```python
from build123d import *

# Parameters (mm, degrees)
BOSS_EXTRUDE1_DEPTH      = 12.7
BOSS_EXTRUDE1_DEPTH_BACK = 19.878167
SKETCH1_W                = 76.2
SKETCH1_H                = 25.4
CUT_EXTRUDE1_DEPTH       = 50.919049703
SKETCH4_R                = 7.9375
BOSS_EXTRUDE2_DEPTH      = 76.2
BOSS_EXTRUDE3_DEPTH      = 10


with BuildPart() as part:
    # Sketch1 → Boss-Extrude1 (new, two sides: drawn at the far end of the back side and taken through both)
    with BuildSketch(Plane.XY.offset(-BOSS_EXTRUDE1_DEPTH_BACK)):
        Rectangle(SKETCH1_W, SKETCH1_H)
    extrude(amount=BOSS_EXTRUDE1_DEPTH + BOSS_EXTRUDE1_DEPTH_BACK)

    # Sketch2 → Cut-Extrude1 (cut, through all)
    with BuildSketch(Plane.XZ.offset(12.7)):
        Polygon((33.097822487, -3.5890835), (28.095644974, -19.878167), (30.299971912, -19.878167), (38.1, -19.878167), (38.1, -5.125190787), align=None)
        Polygon((38.1, 12.7), (33.097822487, -3.5890835), (38.1, -5.125190787), align=None)
        with BuildLine():
            Line((28.095644974, -19.878167), (-38.1, -19.878167))
            Line((-38.1, -19.878167), (-38.1, 2.7))
            Line((-38.1, 2.7), (-9.105646135, 2.7))
            add(Edge.make_bspline(
                [(28.095644974, -19.878167), (23.262476233, -19.878167), (13.759725723, -18.38827049), (5.19295176, 1.21010349), (-4.185142014, 2.7), (-9.105646135, 2.7)],
                knots=[0, 0, 0, 0, 0.311689084, 0.688310916, 1, 1, 1, 1], degree=3))
        make_face()
    extrude(amount=-CUT_EXTRUDE1_DEPTH, mode=Mode.SUBTRACT)

    # Sketch4 → Boss-Extrude2 (add)
    with BuildSketch(Plane(origin=(31.252760971, 0, -9.59733911), x_dir=(-0.2935578385035089, 0, -0.95594131381228), z_dir=(0.95594131381228, 0, -0.2935578385035089))):
        with Locations((-2.530674188, 0)):
            Circle(SKETCH4_R)
    extrude(amount=BOSS_EXTRUDE2_DEPTH)

    # Sketch5 → Boss-Extrude3 (add)
    with BuildSketch(Plane(origin=(0, 0, 2.7), x_dir=(-1, 0, 0), z_dir=(0, 0, -1))):
        Polygon((9.105646135, -12.7), (28.322642206, -26.407350084), (38.1, -12.7), align=None)
        Polygon((38.1, -12.7), (56.217643925, 12.7), (38.1, 12.7), align=None)
        Polygon((16.319736518, -17.845760662), (21.108551823, -21.261589422), (19.992545993, -32.851753107), (5.724357418, -22.674353105), align=None)
    extrude(amount=-BOSS_EXTRUDE3_DEPTH)


solid = part.part
```
For this review, take the finished solid that the model builds, in its own axes (mm). A direction names the side the tool comes from. Give positions to 0.01 mm unless a question says otherwise; leave off trailing zeros. Order: outer loops, then holes, each group sorted by start corner. A loop starts at its lowest first (then second) coordinate and runs counter-clockwise, first axis right, second up.
1) For faces 4 (the face through (-24.67, -23.8, 7.63)), 5 (the face through (-10.948, -20.294, 7.63)), 6 (the face through (34.28, -3, 0.26)), list the 3-axis set-ups (+Z, -Z, +X, -X, +Y, -Y) from which the entire face can be reached by the end or side of a thin tool; tool diameter is ignored.
2) Wall thickness on line 1 (Z direction, x = -29.5, y = -16); line 2 (Y direction, x = 4, z = 2); line 3 (Z direction, x = 22, y = 7.5): over which ranges is each line inside the solid? List them lowest first.
3) Take a section at B-B (y = -30). Give the boundary of the cut face in (x, z).
4) Insertion check: pin 1 (1 mm diameter, centred on y = -7.5, z = -15, fed in from -X); pin 2 (10 mm diameter, centred on x = -27.5, y = -22, fed in from -Z); pin 3 (8 mm diameter, centred on y = -16.5, z = -22, fed in from -X); pin 4 (2 mm diameter, centred on x = 28, y = 3, fed in from -Z). Each pin has a flat end and moves straight along its axis. Give the tip position at first contact, or say it passes through.
5) The part is to be moulded in two halves that separate along X. For faces 1 (the face through (-20.558, -26.976, 7.63)), 2 (the face through (1, 12.7, 3)), 3 (the face through (-12.662, -15.237, 7.63)), say which applies: released by +X, released by -X, zero draft, split by the parting line, or undercut.
6) Take a section at A-A (z = 4.5). Give the boundary of the cut face in (x, y).
7) Take a section at C-C (x = -33). Give the boundary of the cut face in (y, z), then the cut area to 4 significant figures.
Derived:
1. face 4: +Z, -Z, -Y
1. face 5: +Z, -Z, +X
1. face 6: none
2. line 1: z = 2.7 to 12.7
2. line 2: y = -12.7 to 12.7
2. line 3: z = -19.33 to 12.7
3. outline: (-20.27, 2.7) - (-15.99, 2.7) - (-15.99, 12.7) - (-20.27, 12.7) - close
4. pin 1: stops at x = 13.83
4. pin 2: stops at z = 2.7
4. pin 3: passes through
4. pin 4: stops at z = -19.88
5. face 1: undercut
5. face 2: zero draft
5. face 3: released by +X
6. outline: (-56.22, 12.7) - (-28.32, -26.41) - (-21.11, -21.26) - (-19.99, -32.85) - (-5.72, -22.67) - (-16.32, -17.85) - (-9.11, -12.7) - (35.58, -12.7) - (35.58, 12.7) - close
7. outline: (-19.85, 2.7) - (12.7, 2.7) - (12.7, 12.7) - (-19.85, 12.7) - close
7. area: 325.5 mm2
